Job drawing, mm, ordinate dimensions from the low corner. One solid piece. A direction names the side the tool comes from. Round coordinates to 2 decimals unless told otherwise and drop trailing zeros. Order: outer loops, then holes, each group sorted by start corner. A loop starts at its lowest first (then second) coordinate and runs counter-clockwise, first axis right, second up. Notation, with made-up numbers: (-12.75, 15) -> (3.25, 15) arc R17 cw to (3.25, 38) -> close; hole circle Ø2 at (70.5, -33). An arc over 180 degrees is marked (long way). Write item = value, one per line.
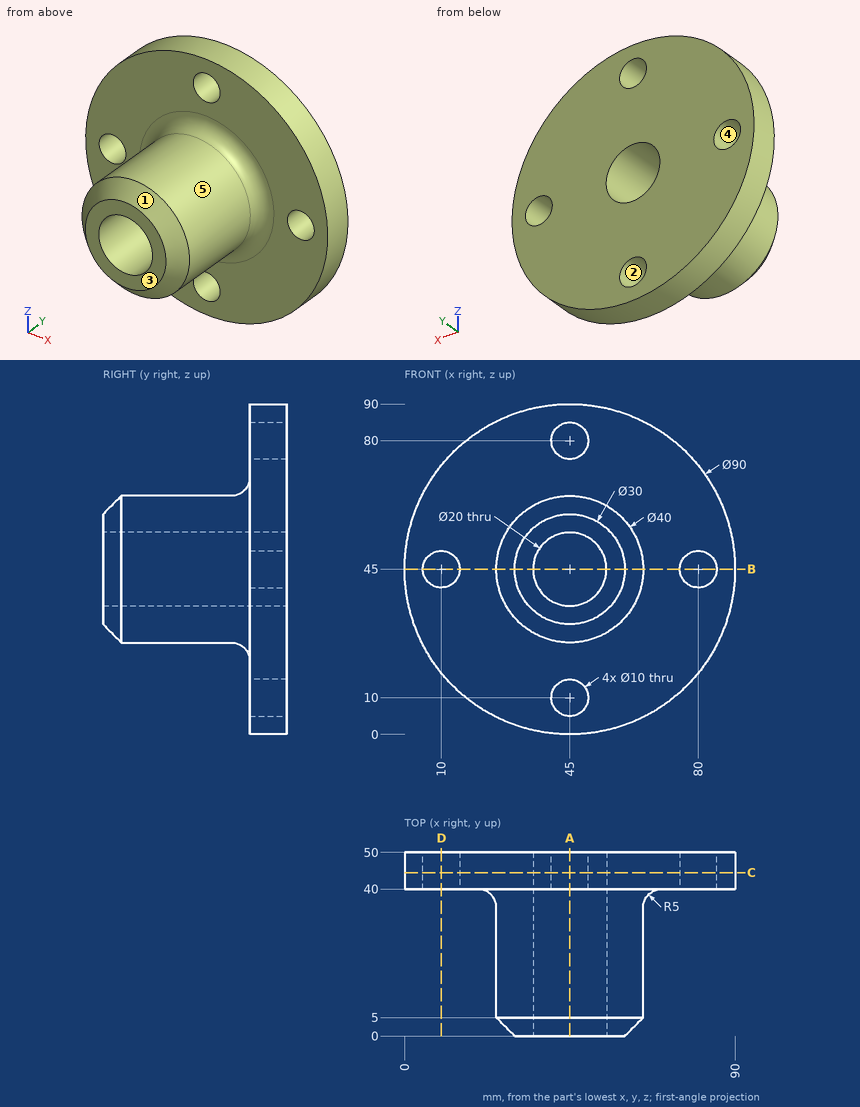
Q1. Cut at D-D, the plane x = 10. List the corners of the cut face in (y, z).
Check values:
outline = (40, 16.72) -> (50, 16.72) -> (50, 40) -> (40, 40) -> close; (40, 50) -> (50, 50) -> (50, 73.28) -> (40, 73.28) -> close
Q2. Probe probe 1 along X at (y, z) = (42.5, 45.5); probe 2 along Y at (x, z) = (73.5, 24); probe 3 along X at (y, z) = (43, 10). List the from-to ranges inside material, lowest first.
Check values:
probe_1 = 0 to 5.03, 14.97 to 35.01, 54.99 to 75.03, 84.97 to 90
probe_2 = 40 to 50
probe_3 = 16.72 to 40, 50 to 73.28
Q3. Which spindle directions (+Z, -Z, +X, -X, +Y, -Y) get a long thin tool onto all of the face, cutting with end or side? Do the marked faces 4 and 5. Say none if no direction does.
Check values:
face_4 = +Y, -Y
face_5 = -Y
Q4. Cut at A-A, the plane x = 45. List the corners of the cut face in (y, z), and give its area (3 significant figures).
Check values:
outline = (0, 30) -> (5, 25) -> (35, 25) arc R5 cw to (40, 20) -> (40, 15) -> (50, 15) -> (50, 35) -> (0, 35) -> close; (0, 55) -> (50, 55) -> (50, 75) -> (40, 75) -> (40, 70) arc R5 cw to (35, 65) -> (5, 65) -> (0, 60) -> close; (40, 0) -> (50, 0) -> (50, 5) -> (40, 5) -> close; (40, 85) -> (50, 85) -> (50, 90) -> (40, 90) -> close
area = 1,290 mm²
Q5. Flat gauge pins, fed straight in: pin 1 (6 mm diameter, centred on y = 17.5, z = 44, fed in from +X); pin 2 (16 mm diameter, centred on x = 45, z = 45, fed in from +Y); pin 3 (6 mm diameter, centred on x = 34, y = 31.5, fed in from +Z); pin 4 (16 mm diameter, centred on x = 10, z = 45, fed in from -Y). Where does each tip first touch, or does it go through?
Check values:
pin_1 = 65
pin_2 = through
pin_3 = 63.33
pin_4 = 40
Q6. Cut at B-B, the plane z = 45. List the corners of the cut face in (x, y).
Check values:
outline = (0, 40) -> (5, 40) -> (5, 50) -> (0, 50) -> close; (15, 40) -> (20, 40) arc R5 cw to (25, 35) -> (25, 5) -> (30, 0) -> (35, 0) -> (35, 50) -> (15, 50) -> close; (55, 0) -> (60, 0) -> (65, 5) -> (65, 35) arc R5 cw to (70, 40) -> (75, 40) -> (75, 50) -> (55, 50) -> close; (85, 40) -> (90, 40) -> (90, 50) -> (85, 50) -> close
Q7. Mould opens along Z. For the marked faces 1, 2 and 3 say: released by +Z, released by -Z, zero draft, split by the parting line, or undercut.
Check values:
face_1 = split by the parting line
face_2 = undercut
face_3 = zero draft
Q8. Cut at C-C, the plane y = 44.5. List the corners of the cut face in (x, z).
Check values:
outline = circle Ø90 at (45, 45); hole circle Ø10 at (10, 45); hole circle Ø20 at (45, 45); hole circle Ø10 at (45, 10); hole circle Ø10 at (45, 80); hole circle Ø10 at (80, 45)
